```python
from build123d import *

# Parameters (mm, degrees)
BOSS_EXTRUDE1_DEPTH                            = 12
CUT_EXTRUDE1_DEPTH                             = 1.5
CUT_EXTRUDE2_DEPTH                             = 8.5
M2X0_4_TAPPED_HOLE1_D                          = 1.6
M2X0_4_TAPPED_HOLE1_DEPTH                      = 6
M2X0_4_TAPPED_HOLE1_CSINK_D                    = 2.05
M2X0_4_TAPPED_HOLE1_CSINK_ANGLE                = 90
M2X0_4_TAPPED_HOLE1_TIP                        = 0.480688495
CSK_FOR_M4_FLAT_HEAD_MACHINE_SCREW2_AT_2_COUNT = 2
CSK_FOR_M4_FLAT_HEAD_MACHINE_SCREW2_AT_2_PITCH = 346
CHAMFER1_SIZE                                  = 1
CUT_EXTRUDE3_DEPTH                             = 10
CUT_EXTRUDE4_DEPTH                             = 10
CUT_EXTRUDE5_DEPTH                             = 0.375
CHAMFER3_SIZE                                  = 0.254


with BuildPart() as part:
    # Sketch1 → Boss-Extrude1 (new body)
    with BuildSketch(Plane(origin=(0, 0, 0), x_dir=(1, 0, 0), z_dir=(0, 1, 0))):
        with BuildLine():
            Line((-5, 109), (-387, 109))
            ThreePointArc((-387, 109), (-391.949747468, 106.949747468), (-394, 102))
            Line((-394, 102), (-394, 5))
            ThreePointArc((-394, 5), (-391.949747468, 0.050252532), (-387, -2))
            Line((-387, -2), (-5, -2))
            ThreePointArc((-5, -2), (-0.050252532, 0.050252532), (2, 5))
            Line((2, 5), (2, 102))
            ThreePointArc((2, 102), (-0.050252532, 106.949747468), (-5, 109))
        make_face()
    extrude(amount=BOSS_EXTRUDE1_DEPTH)

    # Sketch2 → Cut-Extrude1 (cut)
    with BuildSketch(Plane(origin=(0, 12, 0), x_dir=(1, 0, 0), z_dir=(0, 1, 0))):
        with BuildLine():
            Line((0, 5), (0, 102))
            ThreePointArc((0, 102), (-1.464466094, 105.535533906), (-5, 107))
            Line((-5, 107), (-387, 107))
            ThreePointArc((-387, 107), (-390.535533906, 105.535533906), (-392, 102))
            Line((-392, 102), (-392, 5))
            ThreePointArc((-392, 5), (-390.535533906, 1.464466094), (-387, 0))
            Line((-387, 0), (-5, 0))
            ThreePointArc((-5, 0), (-1.464466094, 1.464466094), (0, 5))
        make_face()
    extrude(amount=-CUT_EXTRUDE1_DEPTH, mode=Mode.SUBTRACT)

    # Sketch3 → Cut-Extrude2 (cut)
    with BuildSketch(Plane(origin=(0, 10.5, 0), x_dir=(1, 0, 0), z_dir=(0, 1, 0))):
        with BuildLine():
            Line((-384, 102.5), (-8, 102.5))
            ThreePointArc((-8, 102.5), (-5.525126266, 101.474873734), (-4.5, 99))
            Line((-4.5, 99), (-4.5, 8))
            ThreePointArc((-4.5, 8), (-5.525126266, 5.525126266), (-8, 4.5))
            Line((-8, 4.5), (-384, 4.5))
            ThreePointArc((-384, 4.5), (-386.474873734, 5.525126266), (-387.5, 8))
            Line((-387.5, 8), (-387.5, 99))
            ThreePointArc((-387.5, 99), (-386.474873734, 101.474873734), (-384, 102.5))
        make_face()
    extrude(amount=-CUT_EXTRUDE2_DEPTH, mode=Mode.SUBTRACT)

    # M2x0.4 Tapped Hole1
    with Locations(Plane(origin=(-388, 10.5, -103), x_dir=(0, 0, 1), z_dir=(0, 1, 0))):
        with Locations((0, 0), (-1.5, 96), (-1.5, 192), (-1.5, 288), (0, 384), (99, 384), (100.5, 288), (100.5, 192), (100.5, 96), (99, 0)):
            CounterSinkHole(M2X0_4_TAPPED_HOLE1_D / 2, M2X0_4_TAPPED_HOLE1_CSINK_D / 2, depth=M2X0_4_TAPPED_HOLE1_DEPTH, counter_sink_angle=M2X0_4_TAPPED_HOLE1_CSINK_ANGLE)
            with Locations((0, 0, -(M2X0_4_TAPPED_HOLE1_DEPTH + M2X0_4_TAPPED_HOLE1_TIP / 2))):  # 118° drill point
                Cone(0, M2X0_4_TAPPED_HOLE1_D / 2, M2X0_4_TAPPED_HOLE1_TIP, mode=Mode.SUBTRACT)

    # Sketch19 → CSK for M4 Flat Head Machine Screw2 (revolve, cut)
    with BuildSketch(Plane(origin=(-369, 2, -84), x_dir=(0, 0, 1), z_dir=(1, 0, 0))):
        Polygon((0, 0), (0, 2), (2.15, 2), (2.15, 1.709665499), (4.1875, 0), align=None)
    csk_for_m4_flat_head_machine_screw2 = revolve(axis=Axis((-369, 8.35, -84), (0, -1, 0)), mode=Mode.SUBTRACT)

    # CSK for M4 Flat Head Machine Screw2 at 2: CSK for M4 Flat Head Machine Screw2 ×2
    with Locations(*[(i * CSK_FOR_M4_FLAT_HEAD_MACHINE_SCREW2_AT_2_PITCH, 0, 0) for i in range(1, CSK_FOR_M4_FLAT_HEAD_MACHINE_SCREW2_AT_2_COUNT)]):
        add(csk_for_m4_flat_head_machine_screw2, mode=Mode.SUBTRACT)

    # Chamfer1
    chamfer1_edges = [part.edges().sort_by_distance(p)[0] for p in [
        (-391.949747468, 12, -106.949747468),
        (-196, 0, -109),
        (-0.050252532, 0, -106.949747468),
        (-394, 12, -53.5),
        (-391.949747468, 12, -0.050252532),
        (-196, 12, 2),
        (-0.050252532, 12, -0.050252532),
        (2, 12, -53.5),
        (-0.050252532, 12, -106.949747468),
        (-196, 12, -109),
        (2, 0, -53.5),
        (-0.050252532, 0, -0.050252532),
        (-196, 0, 2),
        (-391.949747468, 0, -0.050252532),
        (-394, 0, -53.5),
        (-391.949747468, 0, -106.949747468),
    ]]
    chamfer(chamfer1_edges, length=CHAMFER1_SIZE)

    # Sketch20 → Cut-Extrude3 (cut)
    with BuildSketch(Plane(origin=(0, 2, 0), x_dir=(1, 0, 0), z_dir=(0, 1, 0))):
        with BuildLine():
            Line((-45.6072, 101.5), (-50.491454659, 106.058681888))
            ThreePointArc((-50.491454659, 106.058681888), (-51.596106449, 106.756177714), (-52.879580912, 107))
            Line((-52.879580912, 107), (-64.120419088, 107))
            ThreePointArc((-64.120419088, 107), (-65.403893551, 106.756177714), (-66.508545341, 106.058681888))
            Line((-66.508545341, 106.058681888), (-71.3928, 101.5))
            Line((-71.3928, 101.5), (-45.6072, 101.5))
        make_face()
    extrude(amount=CUT_EXTRUDE3_DEPTH, mode=Mode.SUBTRACT)

    # Sketch21 → Cut-Extrude4 (cut)
    with BuildSketch(Plane(origin=(0, 0, -109), x_dir=(-1, 0, 0), z_dir=(0, 0, -1))):
        with BuildLine():
            Line((55.100019088, 5.5), (61.900019088, 5.5))
            ThreePointArc((61.900019088, 5.5), (62.783902564, 5.133883476), (63.150019088, 4.25))
            Line((63.150019088, 4.25), (63.150019088, 3.25))
            ThreePointArc((63.150019088, 3.25), (62.783902564, 2.366116524), (61.900019088, 2))
            Line((61.900019088, 2), (55.100019088, 2))
            ThreePointArc((55.100019088, 2), (54.216135611, 2.366116524), (53.850019088, 3.25))
            Line((53.850019088, 3.25), (53.850019088, 4.25))
            ThreePointArc((53.850019088, 4.25), (54.216135611, 5.133883476), (55.100019088, 5.5))
        make_face()
    extrude(amount=-CUT_EXTRUDE4_DEPTH, mode=Mode.SUBTRACT)

    # Sketch22 → Cut-Extrude5 (cut)
    with BuildSketch(Plane(origin=(0, 0, -109), x_dir=(-1, 0, 0), z_dir=(0, 0, -1))):
        with BuildLine():
            Line((51.500019088, -6.125), (51.500019088, 4.7))
            ThreePointArc((51.500019088, 4.7), (52.429955058, 6.94506403), (54.675019088, 7.875))
            Line((54.675019088, 7.875), (62.325019088, 7.875))
            ThreePointArc((62.325019088, 7.875), (64.570083118, 6.94506403), (65.500019088, 4.7))
            Line((65.500019088, 4.7), (65.500019088, -6.125))
            Line((65.500019088, -6.125), (51.500019088, -6.125))
        make_face()
    extrude(amount=-CUT_EXTRUDE5_DEPTH, mode=Mode.SUBTRACT)

    # Chamfer3
    chamfer3_edges = [part.edges().sort_by_distance(p)[0] for p in [
        (-54.216135611, 2.366116524, -108.625),
        (-58.500019088, 5.5, -108.625),
        (-54.216135611, 5.133883476, -108.625),
        (-53.850019088, 3.75, -108.625),
        (-58.500019088, 2, -108.625),
        (-62.783902564, 2.366116524, -108.625),
        (-63.150019088, 3.75, -108.625),
        (-62.783902564, 5.133883476, -108.625),
    ]]
    chamfer(chamfer3_edges, length=CHAMFER3_SIZE)


solid = part.part
```
Could you check a few things on this model? Use its own coordinates, in mm. A direction names the side the tool comes from. Give positions to 0.01 mm unless a question says otherwise; leave off trailing zeros. Loops run counter-clockwise (first coordinate to the right, second up) from the corner with the lowest first, then second, coordinate; pieces in that order, holes last. Notation, with made-up numbers: (77, 27.5) - (86, 27.5) arc R23 ccw to (86, 48.5) - close; hole circle Ø3 at (-9.5, -33.75). An arc over 180 degrees is marked (long way). Use one line per item in the form item = value.
1. I want a section at B-B (x = -164). Please give me the cut outline in (y, z), and give its area (4 significant figures).
Response values:
outline = (0, -108) - (1, -109) - (11, -109) - (12, -108) - (12, -107) - (10.5, -107) - (10.5, -102.5) - (2, -102.5) - (2, -4.5) - (10.5, -4.5) - (10.5, 0) - (12, 0) - (12, 1) - (11, 2) - (1, 2) - (0, 1) - close
area = 336.5 mm²
2. I need wall thicknesses on probe 1 along Z at (x, y) = (-292, 9.15); probe 2 along Z at (x, y) = (-4, 8.6); probe 3 along X at (y, z) = (8, -70.5). Which ranges of each line are inside material? Lowest first, please.
Response values:
probe_1 = -109 to -105.3, -103.7 to -102.5, -4.5 to -3.3, -1.7 to 2
probe_2 = -108.93 to -103.8, -102.2 to -4.8, -3.2 to 1.93
probe_3 = -394 to -387.5, -4.5 to 2
3. I'm going to push flat-ended pins straight in: pin 1 Ø2 at (x, z) = (-100, -104.5) entering from +Y (3 decimals); pin 2 Ø0.8 at (y, z) = (11.5, -38) entering from +X; pin 3 Ø1.1 at (y, z) = (3.5, -107.5) entering from +X. Where does each tip first touch, or does it pass through?
Response values:
pin_1 = 10.475
pin_2 = 1.9
pin_3 = -0.05
4. I want a section at A-A (z = -53). Please give me the cut outline in (x, y).
Response values:
outline = (-394, 1) - (-393, 0) - (1, 0) - (2, 1) - (2, 11) - (1, 12) - (0, 12) - (0, 10.5) - (-4.5, 10.5) - (-4.5, 2) - (-387.5, 2) - (-387.5, 10.5) - (-392, 10.5) - (-392, 12) - (-393, 12) - (-394, 11) - close
5. On a 3-axis mill with a long thin cutter (end or side, diameter ignored), from which of +Z, -Z, +X, -X, +Y, -Y can I reach the whole of each face in a straight line? I mean faces 1 (the face through (-391.31, 11.84, -106.4)), 2 (the face through (-211, 10.5, -2)). Say none if no direction works.
Response values:
face_1 = -Z, -X, +Y
face_2 = +Y
6. Thinking about a two-plate mould opening in Z: for faces 3 (the face through (2, 6, -53)), 4 (the face through (-392, 5.9, -0.1)), 5 (the face through (-0.6, 11.84, -106.31)), 6 (the face through (-229, 6, -102.5)), which applies, released by +Z, released by -Z, zero draft, split by the parting line, or undercut?
Response values:
face_3 = zero draft
face_4 = released by +Z
face_5 = released by -Z
face_6 = undercut
